The drawing under review shows one solid part. Ordinate dimensions are in mm from its lowest x, y, z. Coordinates: 2 decimals unless noted, no trailing zeros. Order: outer loops, then holes, each group sorted by start corner. A loop starts at its lowest first (then second) coordinate and runs counter-clockwise, first axis right, second up. Notation, with made-up numbers: (-7, -31.5) -> (6, -31.5) arc R26 ccw to (6, -16.5) -> close; hole circle Ø6 at (6.5, 12.5). An arc over 180 degrees is marked (long way). Write item = value, one per line.
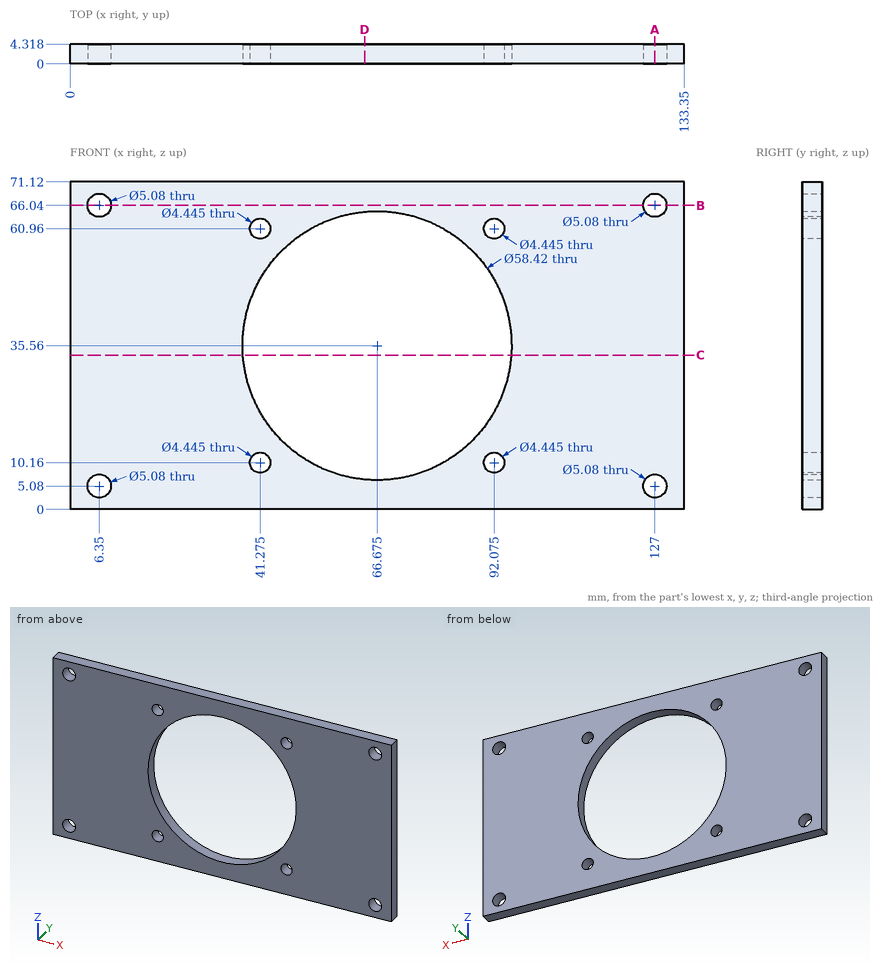
(1) Insertion check: pin 1 (3.5 mm diameter, centred on x = 41.275, z = 60.96, fed in from -Y); pin 2 (7 mm diameter, centred on x = 41.275, z = 10.16, fed in from +Y). Each pin has a flat end and moves straight along its axis. Give the tip position at first contact, or say it passes through.
Report:
pin_1 = through
pin_2 = 4.32
(2) We need section B-B (z = 66.04). Write out the cut boundary in (x, y).
Report:
outline = (0, 0) -> (3.81, 0) -> (3.81, 4.32) -> (0, 4.32) -> close; (8.89, 0) -> (124.46, 0) -> (124.46, 4.32) -> (8.89, 4.32) -> close; (129.54, 0) -> (133.35, 0) -> (133.35, 4.32) -> (129.54, 4.32) -> close
(3) We need section A-A (x = 127). Write out the cut boundary in (y, z), and give its area (3 significant figures).
Report:
outline = (0, 0) -> (4.32, 0) -> (4.32, 2.54) -> (0, 2.54) -> close; (0, 7.62) -> (4.32, 7.62) -> (4.32, 63.5) -> (0, 63.5) -> close; (0, 68.58) -> (4.32, 68.58) -> (4.32, 71.12) -> (0, 71.12) -> close
area = 263 mm²
(4) We need section D-D (x = 64). Write out the cut boundary in (y, z).
Report:
outline = (0, 0) -> (4.32, 0) -> (4.32, 6.47) -> (0, 6.47) -> close; (0, 64.65) -> (4.32, 64.65) -> (4.32, 71.12) -> (0, 71.12) -> close
(5) For L1, parallel to X at y = 3.45, z = 10.16; L2, parallel to Z at x = 93, y = 0.2; L3, parallel to X at y = 1.3, z = 5.08, list the stretches that pass through material, from the lowest coordinate up.
Report:
L1 = 0 to 39.05, 43.5 to 52.25, 81.1 to 89.85, 94.3 to 133.35
L2 = 0 to 8.14, 12.18 to 22.9, 48.22 to 58.94, 62.98 to 71.12
L3 = 0 to 3.81, 8.89 to 124.46, 129.54 to 133.35
(6) We need section C-C (z = 33.5). Write out the cut boundary in (x, y), and give its area (3 significant figures).
Report:
outline = (0, 0) -> (37.54, 0) -> (37.54, 4.32) -> (0, 4.32) -> close; (95.81, 0) -> (133.35, 0) -> (133.35, 4.32) -> (95.81, 4.32) -> close
area = 324 mm²
